Read the model definition and answer for the solid it produces. Units are mm, in the model's axes. A direction names the side the tool comes from. Coordinates: 2 decimals unless noted, no trailing zeros. Order: outer loops, then holes, each group sorted by start corner. A loop starts at its lowest first (then second) coordinate and runs counter-clockwise, first axis right, second up. Notation, with made-up numbers: M 65.5,39 L 96.5,39 A21 ccw 96.5,68 Z; hole C 34.25,-22 d11. An arc over 180 degrees is marked long. Put each result on its own line as item: value.
from build123d import *

# Parameters (mm, degrees)
SKETCH_1_R          = 3.9
EXTRUDE_1_DEPTH     = 4
SKETCH_2_R          = 6
EXTRUDE_2_DEPTH     = 2
SKETCH_6_R          = 2.9
EXTRUDE_3_DEPTH     = 7.6
SKETCH_3_R          = 1.6
CUT_EXTRUDE_1_DEPTH = 17.029971928
SKETCH_4_R          = 3
CUT_EXTRUDE_2_DEPTH = 3.5


with BuildPart() as part:
    # 草图1 → 凸台-拉伸1 (new body)
    with BuildSketch(Plane(origin=(0, 0, 0), x_dir=(1, 0, 0), z_dir=(0, 1, 0))):
        with Locations(Location((0, 0, 0), (0, 0, 270))):
            Circle(SKETCH_1_R)
    extrude(amount=EXTRUDE_1_DEPTH)

    # 草图2 → 凸台-拉伸2 (add)
    with BuildSketch(Plane(origin=(0, 4, 0), x_dir=(1, 0, 0), z_dir=(0, 1, 0))):
        with Locations(Location((0, 0, 0), (0, 0, 270))):
            Circle(SKETCH_2_R)
    extrude(amount=EXTRUDE_2_DEPTH)

    # 草图6 → 凸台-拉伸3 (add)
    with BuildSketch(Plane.XZ):
        with Locations(Location((0, 0, 0), (0, 0, 90))):
            Circle(SKETCH_6_R)
    extrude(amount=EXTRUDE_3_DEPTH)

    # 草图3 → 切除-拉伸1 (cut, through all)
    with BuildSketch(Plane(origin=(0, 6, 0), x_dir=(1, 0, 0), z_dir=(0, 1, 0))):
        with Locations(Location((0, 0, 0), (0, 0, 270))):
            Circle(SKETCH_3_R)
    extrude(amount=-CUT_EXTRUDE_1_DEPTH, mode=Mode.SUBTRACT)

    # 草图4 → 切除-拉伸2 (cut)
    with BuildSketch(Plane(origin=(0, 6, 0), x_dir=(1, 0, 0), z_dir=(0, 1, 0))):
        with Locations(Location((0, 0, 0), (0, 0, 270))):
            Circle(SKETCH_4_R)
    extrude(amount=-CUT_EXTRUDE_2_DEPTH, mode=Mode.SUBTRACT)


solid = part.part
Q1. Find section B-B on z = 0. Write down the section's boundary in (x, y).
Answers below:
outline: M -6,4 L -3.9,4 L -3.9,0 L -2.9,0 L -2.9,-7.6 L -1.6,-7.6 L -1.6,2.5 L -3,2.5 L -3,6 L -6,6 Z; M 1.6,-7.6 L 2.9,-7.6 L 2.9,0 L 3.9,0 L 3.9,4 L 6,4 L 6,6 L 3,6 L 3,2.5 L 1.6,2.5 Z
Q2. Find section D-D on x = 3.5. Write down the section's boundary in (y, z), plus the area to 3 significant figures.
Answers below:
outline: M 0,-1.72 L 4,-1.72 L 4,-4.87 L 6,-4.87 L 6,4.87 L 4,4.87 L 4,1.72 L 0,1.72 Z
area: 33.3 mm^2
Q3. A tool of negligible diameter and unlimited length cuts with its end or side. For faces 1 (the face through (1.25, -7.6, 1.25)), 2 (the face through (0.9, 4.27, 2.86)), 3 (the face through (3, 0, -1)), from which of +Z, -Z, +X, -X, +Y, -Y can it reach the whole face along a straight path? Write none if from no direction.
Answers below:
face 1: +Z, -Z, +X, -X, -Y
face 2: +Y
face 3: -Y
Q4. For a pull along Z with two mould halves and no side action, classify faces 4 (the face through (-0.1, -3.7, -2.9)), 5 (the face through (-4, 4, 1)), 6 (the face through (-0.97, -2.48, -1.27)) as +Z half, -Z half, draft (parallel to the pull), parting line (faces both ways), or undercut.
Answers below:
face 4: parting line
face 5: draft
face 6: undercut
Q5. Find section A-A on x = 0. Write down the section's boundary in (y, z).
Answers below:
outline: M -7.6,-2.9 L 0,-2.9 L 0,-3.9 L 4,-3.9 L 4,-6 L 6,-6 L 6,-3 L 2.5,-3 L 2.5,-1.6 L -7.6,-1.6 Z; M -7.6,1.6 L 2.5,1.6 L 2.5,3 L 6,3 L 6,6 L 4,6 L 4,3.9 L 0,3.9 L 0,2.9 L -7.6,2.9 Z
Q6. Given pin 1 (5 mm diameter, centred on x = -2.5, y = -4, fed in from -Z); pin 2 (1.5 mm diameter, centred on y = 2.5, z = -2.5, fed in from -X); pin 3 (2 mm diameter, centred on x = -4, z = -4.5, fed in from -Y), each flat-ended and moving along its own axis, determine where each tip first touches the part or whether it passes through.
Answers below:
pin 1: stops at z = -2.9
pin 2: stops at x = -3.49
pin 3: stops at y = 4
Q7. Find section C-C on y = 3.5. Write down the section's boundary in (x, z), plus the area to 3 significant figures.
Answers below:
outline: C 0,0 d7.8; hole C 0,0 d6
area: 19.5 mm^2
Q8. Consider line 1 along X through (y, z) = (-3, 0); line 2 along X through (y, z) = (4.7, 0); line 3 along Y through (x, z) = (3.25, 2.25). Determine where each line is inside the solid, lowest interval first.
Answers below:
line 1: x = -2.9 to -1.6, 1.6 to 2.9
line 2: x = -6 to -3, 3 to 6
line 3: y = 4 to 6
